The listing builds one solid part. Answer for the finished solid, in the listing's coordinates (mm). A direction names the side the tool comes from. Round coordinates to 2 decimals unless told otherwise and drop trailing zeros. Write each loop counter-clockwise with the first axis right and the second up, starting at its lowest first coordinate (ties: lowest second). Pieces come first, ordered by that corner, then holes. Notation, with made-up numbers: M 87.25,65.5 L 140.25,65.5 A13 cw 140.25,88.5 Z; hole C 73.25,3.25 d8. An arc over 180 degrees is marked long. Put each result on its own line as item: value. Start each with the question number.
```python
from build123d import *

# Parameters (mm, degrees)
SKETCH1_W                                = 157.01375
SKETCH1_H                                = 100.80625
BOSS_EXTRUDE1_DEPTH                      = 10.16
SKETCH2_W                                = 144.31375
SKETCH2_H                                = 88.10625
CUT_EXTRUDE1_DEPTH                       = 3.81
SKETCH3_R                                = 1.373000048
BOSS_EXTRUDE2_DEPTH                      = 13.208
SKETCH4_R                                = 1.905
SKETCH4_W                                = 38.820000042
SKETCH4_H                                = 30.86
BOSS_EXTRUDE3_DEPTH                      = 3.556
SKETCH5_W                                = 140.45073311
SKETCH5_H                                = 20.997286457
CUT_EXTRUDE2_DEPTH                       = 61.722
SKETCH6_W                                = 3.175
SKETCH6_H                                = 3.175
BOSS_EXTRUDE4_DEPTH                      = 6.985
SKETCH7_W                                = 1.5875
SKETCH7_H                                = 1.5875
CUT_EXTRUDE3_DEPTH                       = 6.985
MIRROR2_COPY_1_SKETCH_W                  = 3.175
MIRROR2_COPY_1_SKETCH_H                  = 3.175
MIRROR2_COPY_1_DEPTH                     = 6.985
MIRROR2_COPY_2_SKETCH_W                  = 1.5875
MIRROR2_COPY_2_SKETCH_H                  = 1.5875
MIRROR2_COPY_2_DEPTH                     = 6.985
CUT_EXTRUDE4_DEPTH                       = 3.175
MIRROR3_AT_THE_SECOND_PLANE_COPY_1_DEPTH = 3.175
FILLET1_R                                = 1.27
SKETCH9_W                                = 23.8125
SKETCH9_H                                = 15.875
BOSS_EXTRUDE5_DEPTH                      = 11.4935
CUT_EXTRUDE5_START                       = -1.5875
SKETCH10_W                               = 9.261227228
SKETCH10_H                               = 18.25625
CUT_EXTRUDE5_DEPTH                       = 13.97
SKETCH12_W                               = 17.78
SKETCH12_H                               = 18.25625
BOSS_EXTRUDE6_DEPTH                      = 3.01625
SKETCH13_W                               = 3.175
SKETCH13_H                               = 8.09625
BOSS_EXTRUDE7_DEPTH                      = 5.08
BOSS_EXTRUDE9_DEPTH                      = 1.5875
SKETCH17_W                               = 25.4
SKETCH17_H                               = 3.81
SKETCH17_W_2                             = 3.81
SKETCH17_H_2                             = 6.35
BOSS_EXTRUDE10_DEPTH                     = 5.36575
SKETCH18_W                               = 19.05
SKETCH18_H                               = 17.414875
SKETCH18_W_2                             = 6.35
BOSS_EXTRUDE11_DEPTH                     = 3.556
SKETCH19_W                               = 13.81125
SKETCH19_H                               = 4.34975
BOSS_EXTRUDE12_DEPTH                     = 6.35
SKETCH21_W                               = 5.794375
SKETCH21_H                               = 6.35
BOSS_EXTRUDE13_DEPTH                     = 10.4775
SKETCH22_W                               = 19.84375
SKETCH22_H                               = 0.79375
CUT_EXTRUDE6_DEPTH                       = 6.12775
SKETCH23_W                               = 1.905
SKETCH23_H                               = 6.35
SKETCH23_W_2                             = 25.4
SKETCH23_H_2                             = 1.905
CUT_EXTRUDE7_DEPTH                       = 5.36575


with BuildPart() as part:
    # Sketch1 → Boss-Extrude1 (new body)
    with BuildSketch(Plane.XY):
        with Locations((-142.135983, -138.289483)):
            Rectangle(SKETCH1_W, SKETCH1_H)
    extrude(amount=BOSS_EXTRUDE1_DEPTH)

    # Sketch2 → Cut-Extrude1 (cut)
    with BuildSketch(Plane(origin=(0, 0, 0), x_dir=(-1, 0, 0), z_dir=(0, 0, -1))):
        with Locations((142.135983, -138.289483)):
            Rectangle(SKETCH2_W, SKETCH2_H)
    extrude(amount=-CUT_EXTRUDE1_DEPTH, mode=Mode.SUBTRACT)

    # Sketch3 → Boss-Extrude2 (add)
    with BuildSketch(Plane(origin=(0, 0, 3.81), x_dir=(-1, 0, 0), z_dir=(0, 0, -1))):
        with Locations((109.299108, -111.990108)):
            Circle(SKETCH3_R)
        with Locations((156.249108, -111.990108)):
            Circle(SKETCH3_R)
        with Locations((156.249108, -136.500108)):
            Circle(SKETCH3_R)
        with Locations((109.299108, -136.500108)):
            Circle(SKETCH3_R)
    extrude(amount=BOSS_EXTRUDE2_DEPTH)

    # Sketch4 → Boss-Extrude3 (add)
    # profile 1 of 3: a face of its own
    with BuildSketch(Plane(origin=(0, 0, 3.81), x_dir=(-1, 0, 0), z_dir=(0, 0, -1))):
        with Locations(Location((109.299108, -111.990108, 0), (0, 0, 180))):
            Circle(SKETCH4_R)
    # profile 2 of 3: a face of its own
    with BuildSketch(Plane(origin=(0, 0, 3.81), x_dir=(-1, 0, 0), z_dir=(0, 0, -1))):
        with Locations(Location((109.299108, -136.500108, 0), (0, 0, 180))):
            Circle(SKETCH4_R)
    # profile 3 of 3: a face of its own
    with BuildSketch(Plane(origin=(0, 0, 3.81), x_dir=(-1, 0, 0), z_dir=(0, 0, -1))):
        Polygon((112.454108, -105.170108), (191.274108, -105.170108), (191.274108, -110.270108), (201.354108, -110.270108), (201.354108, -143.270108), (112.454108, -143.270108), align=None)
        with Locations((135.039108021, -124.245108)):
            Rectangle(SKETCH4_W, SKETCH4_H, mode=Mode.SUBTRACT)
    extrude(amount=BOSS_EXTRUDE3_DEPTH)

    # Sketch5 → Cut-Extrude2 (cut)
    with BuildSketch(Plane(origin=(0, -87.886358, 0), x_dir=(1, 0, 0), z_dir=(0, 1, 0))):
        with Locations((-140.972363451, 12.879893229)):
            Rectangle(SKETCH5_W, SKETCH5_H)
    extrude(amount=-CUT_EXTRUDE2_DEPTH, mode=Mode.SUBTRACT)

    # Sketch6 → Boss-Extrude4 (add)
    with BuildSketch(Plane(origin=(0, 0, 3.81), x_dir=(-1, 0, 0), z_dir=(0, 0, -1))):
        with Locations((71.566608, -180.755108)):
            Rectangle(SKETCH6_W, SKETCH6_H)
    boss_extrude4 = extrude(amount=BOSS_EXTRUDE4_DEPTH)

    # Sketch7 → Cut-Extrude3 (cut)
    with BuildSketch(Plane(origin=(0, 0, -3.175), x_dir=(-1, 0, 0), z_dir=(0, 0, -1))):
        with Locations((72.360358, -179.961358)):
            Rectangle(SKETCH7_W, SKETCH7_H)
    cut_extrude3 = extrude(amount=-CUT_EXTRUDE3_DEPTH, mode=Mode.SUBTRACT)

    # Mirror1: Boss-Extrude4, Cut-Extrude3 across plane
    add(boss_extrude4.mirror(Plane(origin=(0, -138.289483, 0), x_dir=(0, 0, 1), z_dir=(0, -1, 0))))
    add(cut_extrude3.mirror(Plane(origin=(0, -138.289483, 0), x_dir=(0, 0, 1), z_dir=(0, -1, 0))), mode=Mode.SUBTRACT)

    # Mirror2: Boss-Extrude4, Cut-Extrude3 across plane
    add(boss_extrude4.mirror(Plane(origin=(-142.135983, 0, 0), x_dir=(0, 0, 1), z_dir=(1, 0, 0))))
    add(cut_extrude3.mirror(Plane(origin=(-142.135983, 0, 0), x_dir=(0, 0, 1), z_dir=(1, 0, 0))), mode=Mode.SUBTRACT)

    # Mirror2 copy 1 sketch → Mirror2 copy 1 (add)
    with BuildSketch(Plane(origin=(-284.271966, -276.578966, 3.81), x_dir=(1, 0, 0), z_dir=(0, 0, -1))):
        with Locations((71.566608, -180.755108)):
            Rectangle(MIRROR2_COPY_1_SKETCH_W, MIRROR2_COPY_1_SKETCH_H)
    extrude(amount=MIRROR2_COPY_1_DEPTH)

    # Mirror2 copy 2 sketch → Mirror2 copy 2 (cut)
    with BuildSketch(Plane(origin=(-284.271966, -276.578966, -3.175), x_dir=(1, 0, 0), z_dir=(0, 0, -1))):
        with Locations((72.360358, -179.961358)):
            Rectangle(MIRROR2_COPY_2_SKETCH_W, MIRROR2_COPY_2_SKETCH_H)
    extrude(amount=-MIRROR2_COPY_2_DEPTH, mode=Mode.SUBTRACT)

    # Sketch8 → Cut-Extrude4 (cut)
    with BuildSketch(Plane(origin=(0, 0, -3.175), x_dir=(-1, 0, 0), z_dir=(0, 0, -1))):
        Polygon((69.979108, -179.167608), (70.1775455, -179.167608), (70.1775455, -182.1441705), (73.154108, -182.1441705), (73.154108, -182.342608), (69.979108, -182.342608), align=None)
    cut_extrude4 = extrude(amount=-CUT_EXTRUDE4_DEPTH, mode=Mode.SUBTRACT)

    # Mirror3: Cut-Extrude4 across plane
    add(cut_extrude4.mirror(Plane(origin=(-142.135983, 0, 0), x_dir=(0, 0, 1), z_dir=(1, 0, 0))), mode=Mode.SUBTRACT)

    # Mirror3 at the second plane: Cut-Extrude4 across plane
    add(cut_extrude4.mirror(Plane(origin=(0, -138.289483, 0), x_dir=(0, 0, 1), z_dir=(0, -1, 0))), mode=Mode.SUBTRACT)

    # Mirror3 at the second plane copy 1 sketc → Mirror3 at the second plane copy 1 (cut)
    with BuildSketch(Plane(origin=(-284.271966, -276.578966, -3.175), x_dir=(1, 0, 0), z_dir=(0, 0, -1))):
        Polygon((69.979108, -179.167608), (70.1775455, -179.167608), (70.1775455, -182.1441705), (73.154108, -182.1441705), (73.154108, -182.342608), (69.979108, -182.342608), align=None)
    extrude(amount=-MIRROR3_AT_THE_SECOND_PLANE_COPY_1_DEPTH, mode=Mode.SUBTRACT)

    # Fillet1
    fillet1_edges = [part.edges().sort_by_distance(p)[0] for p in [
        (-220.642858, -138.289483, 10.16),
        (-142.135983, -188.692608, 10.16),
        (-63.629108, -138.289483, 10.16),
        (-63.629108, -188.692608, 5.08),
        (-220.642858, -188.692608, 5.08),
        (-220.642858, -87.886358, 5.08),
        (-63.629108, -87.886358, 5.08),
        (-142.135983, -87.886358, 10.16),
    ]]
    fillet(fillet1_edges, radius=FILLET1_R)

    # Sketch9 → Boss-Extrude5 (add)
    with BuildSketch(Plane(origin=(0, 0, 3.81), x_dir=(-1, 0, 0), z_dir=(0, 0, -1))):
        with Locations((192.464733, -166.070733)):
            Rectangle(SKETCH9_W, SKETCH9_H)
    extrude(amount=BOSS_EXTRUDE5_DEPTH)

    # Sketch10 → Cut-Extrude5 (cut)
    with BuildSketch(Plane(origin=(-63.629108, 0, 0), x_dir=(0, 0, -1), z_dir=(1, 0, 0)).offset(CUT_EXTRUDE5_START)):
        with Locations((3.836863614, -138.289483)):
            Rectangle(SKETCH10_W, SKETCH10_H)
    extrude(amount=-CUT_EXTRUDE5_DEPTH, mode=Mode.SUBTRACT)

    # Sketch12 → Boss-Extrude6 (add)
    with BuildSketch(Plane(origin=(0, 0, 3.81), x_dir=(-1, 0, 0), z_dir=(0, 0, -1))):
        with Locations((78.869108, -138.289483)):
            Rectangle(SKETCH12_W, SKETCH12_H)
    extrude(amount=BOSS_EXTRUDE6_DEPTH)

    # Sketch13 → Boss-Extrude7 (add)
    with BuildSketch(Plane(origin=(0, 0, 3.81), x_dir=(-1, 0, 0), z_dir=(0, 0, -1))):
        with Locations((93.262857978, -138.289483)):
            Rectangle(SKETCH13_W, SKETCH13_H)
    extrude(amount=BOSS_EXTRUDE7_DEPTH)

    # Sketch14 → Boss-Extrude9 (add)
    with BuildSketch(Plane(origin=(-63.629108, 0, 0), x_dir=(0, 0, -1), z_dir=(1, 0, 0))):
        with BuildLine():
            Line((0, -129.288357934), (0, -135.446608))
            ThreePointArc((0, -135.446608), (0.502861016, -134.232594116), (1.7168749, -133.7297331))
            Line((1.7168749, -133.7297331), (1.7168749, -129.288357934))
            Line((1.7168749, -129.288357934), (0, -129.288357934))
        make_face()
        with BuildLine():
            Line((0, -147.290608064), (1.7168749, -147.290608064))
            Line((1.7168749, -147.290608064), (1.7168749, -142.9434829))
            ThreePointArc((1.7168749, -142.9434829), (0.502861016, -142.440621884), (0, -141.226608))
            Line((0, -141.226608), (0, -147.290608064))
        make_face()
    extrude(amount=-BOSS_EXTRUDE9_DEPTH)

    # Sketch17 → Boss-Extrude10 (add)
    with BuildSketch(Plane(origin=(0, 0, 3.81), x_dir=(-1, 0, 0), z_dir=(0, 0, -1))):
        with Locations((155.158483, -172.103233)):
            Rectangle(SKETCH17_W, SKETCH17_H)
        with Locations((155.158483, -150.878358)):
            Rectangle(SKETCH17_W, SKETCH17_H)
        with Locations((175.6769205, -161.4907955)):
            Rectangle(SKETCH17_W_2, SKETCH17_H_2)
        with Locations((134.6400455, -161.4907955)):
            Rectangle(SKETCH17_W_2, SKETCH17_H_2)
    extrude(amount=BOSS_EXTRUDE10_DEPTH)

    # Sketch18 → Boss-Extrude11 (add)
    with BuildSketch(Plane(origin=(0, 0, 3.81), x_dir=(-1, 0, 0), z_dir=(0, 0, -1))):
        with Locations((146.0700455, -161.4907955)):
            Rectangle(SKETCH18_W, SKETCH18_H)
        with Locations((170.5969205, -161.4907955)):
            Rectangle(SKETCH18_W_2, SKETCH18_H)
    extrude(amount=BOSS_EXTRUDE11_DEPTH)

    # Sketch19 → Boss-Extrude12 (add)
    with BuildSketch(Plane.XZ.offset(188.692608)):
        with Locations((-157.943647906, -2.174875)):
            Rectangle(SKETCH19_W, SKETCH19_H)
    extrude(amount=-BOSS_EXTRUDE12_DEPTH)

    # Sketch21 → Boss-Extrude13 (add)
    with BuildSketch(Plane(origin=(0, 0, 0), x_dir=(-1, 0, 0), z_dir=(0, 0, -1))):
        with Locations((148.140835406, -185.517608)):
            Rectangle(SKETCH21_W, SKETCH21_H)
        with Locations((167.746460406, -185.517608)):
            Rectangle(SKETCH21_W, SKETCH21_H)
    extrude(amount=BOSS_EXTRUDE13_DEPTH)

    # Sketch22 → Cut-Extrude6 (cut)
    with BuildSketch(Plane(origin=(0, 0, -10.4775), x_dir=(-1, 0, 0), z_dir=(0, 0, -1))):
        with Locations((157.943647906, -185.517608)):
            Rectangle(SKETCH22_W, SKETCH22_H)
    extrude(amount=-CUT_EXTRUDE6_DEPTH, mode=Mode.SUBTRACT)

    # Sketch23 → Cut-Extrude7 (cut)
    with BuildSketch(Plane(origin=(0, 0, -1.55575), x_dir=(-1, 0, 0), z_dir=(0, 0, -1))):
        with Locations((133.6875455, -161.4907955)):
            Rectangle(SKETCH23_W, SKETCH23_H)
        with Locations((155.158483, -173.055733)):
            Rectangle(SKETCH23_W_2, SKETCH23_H_2)
        with Locations((176.6294205, -161.4907955)):
            Rectangle(SKETCH23_W, SKETCH23_H)
        with Locations((155.158483, -149.925858)):
            Rectangle(SKETCH23_W_2, SKETCH23_H_2)
    extrude(amount=-CUT_EXTRUDE7_DEPTH, mode=Mode.SUBTRACT)


solid = part.part
```
Item 1: Which of the six approach directions +Z, -Z, +X, -X, +Y, -Y give full straight-line access (tool end or side, diameter ignored) to faces 1 (the flat face through (-72, -182.144, -2)), 2 (the flat face through (-192, -174.008, -2)), 3 (the flat face through (-192, -166, -7.683)), 4 (the flat face through (-213, -94.435, -2))?
Item 2: Determine the mould class of faces 5 (the flat face through (-70.178, -96, -2)), 6 (the flat face through (-91.675, -138, 1)), 7 (the flat face through (-214.094, -181, -2)) for opening direction X: released by +X, released by -X, zero draft, split by the parting line, or undercut.
Item 3: Flat-ended cylindrical pins translate along their axes: pin 1 (5 mm diameter, centred on x = -138.5, y = -104.5, fed in from -Z); pin 2 (1.4 mm diameter, centred on x = -155.5, y = -112.5, fed in from -Z); pin 3 (1.3 mm diameter, centred on x = -214, z = -0.5, fed in from +Y); pin 4 (1.5 mm diameter, centred on x = -185, y = -158.5, fed in from -Z). Find the tip coordinate at first contact, or state that the pin passes through.
Item 4: Section C-C (x = -207) is taken. Give the vertices of the cut face in (y, z), and give its area (3 significant figures).
Item 5: Consider line 1 along Y through (x, z) = (-77, 2.75); line 2 along X through (y, z) = (-132, 3.5); line 3 along X through (y, z) = (-153, 0.5). Determine where each line is inside the solid, lowest interval first. Write a range as [from, to].
Item 6: Section B-B (y = -132) is taken. Give the vertices of the cut face in (x, z).
Item 7: Section D-D (x = -139.5) is taken. Give the vertices of the cut face in (y, z), and give its area (3 significant figures).
Item 8: Section A-A (x = -185) is taken. Give the vertices of the cut face in (y, z).
Output values:
1. face 1: -Z, +X, -X, -Y
1. face 2: -Z
1. face 3: -Z, +X, -X, +Y, -Y
1. face 4: -Z, +X, -X, +Y
2. face 5: released by +X
2. face 6: undercut
2. face 7: released by -X
3. pin 1: stops at z = 0.25
3. pin 2: stops at z = -2.38
3. pin 3: stops at y = -87.89
3. pin 4: stops at z = -7.68
4. outline: M -188.69,0 L -182.34,0 L -182.34,3.81 L -94.24,3.81 L -94.24,0 L -87.89,0 L -87.89,8.89 A1.27 ccw -89.16,10.16 L -187.42,10.16 A1.27 ccw -188.69,8.89 Z
4. area: 688 mm^2
5. line 1: y = [-188.69, -182.34], [-147.42, -129.16], [-94.24, -87.89]
5. line 2: x = [-220.64, -214.29], [-201.35, -154.45], [-115.63, -112.45], [-87.76, -63.63]
5. line 3: x = [-220.64, -214.29], [-173.77, -167.42], [-155.6, -136.55], [-69.98, -63.63]
6. outline: M -220.64,0 L -214.29,0 L -214.29,3.81 L -201.35,3.81 L -201.35,0.25 L -154.45,0.25 L -154.45,3.81 L -115.63,3.81 L -115.63,0.25 L -112.45,0.25 L -112.45,3.81 L -87.76,3.81 L -87.76,0.79 L -65.22,0.79 L -65.22,-1.72 L -63.63,-1.72 L -63.63,8.89 A1.27 ccw -64.9,10.16 L -219.37,10.16 A1.27 ccw -220.64,8.89 Z
7. outline: M -188.69,0 L -182.34,0 L -182.34,3.81 L -170.2,3.81 L -170.2,0.25 L -152.78,0.25 L -152.78,3.81 L -143.27,3.81 L -143.27,0.25 L -139.68,0.25 L -139.68,3.81 L -108.82,3.81 L -108.82,0.25 L -105.17,0.25 L -105.17,3.81 L -94.24,3.81 L -94.24,0 L -87.89,0 L -87.89,8.89 A1.27 ccw -89.16,10.16 L -187.42,10.16 A1.27 ccw -188.69,8.89 Z
7. area: 775 mm^2
8. outline: M -188.69,0 L -182.34,0 L -182.34,3.81 L -174.01,3.81 L -174.01,-7.68 L -158.13,-7.68 L -158.13,3.81 L -143.27,3.81 L -143.27,0.25 L -105.17,0.25 L -105.17,3.81 L -94.24,3.81 L -94.24,0 L -87.89,0 L -87.89,8.89 A1.27 ccw -89.16,10.16 L -187.42,10.16 A1.27 ccw -188.69,8.89 Z
